CAD build for the part. Positions are in the model's coordinates, mm. Round coordinates to 2 decimals unless told otherwise and drop trailing zeros. Write each loop counter-clockwise with the first axis right and the second up, starting at its lowest first coordinate (ties: lowest second). Pieces come first, ordered by that corner, then holes. Notation, with made-up numbers: (5.25, -3.5) - (31.25, -3.5) arc R31 cw to (31.25, 34.5) - close; hole circle Ø4 at (-8.75, 86.25). An arc over 180 degrees is marked (long way). Use one line per item in the form item = value. Start each with the question number.
Item 1: Pin check, flat tip, straight feed: pin 1 (6 mm diameter, centred on x = 8, y = -19, fed in from +Z). Stop position of the tip, or through.
Item 2: Band-saw the part on C-C, the plane x = -34. List the corners of the cut face in (y, z), and give its area (3 significant figures).
Item 3: Drill centre lines: L1, parallel to X at y = -3.5, z = 9; L2, parallel to Y at x = 0.5, z = 6; L3, parallel to Z at x = -29.5, y = 23.5. Where is each one in solid material? Low to high.
Item 4: Band-saw the part on A-A, the plane z = 7.25. List the corners of the cut face in (x, y), and give its area (3 significant figures).
Item 5: Band-saw the part on B-B, the plane y = 60. List the corners of the cut face in (x, z).
from build123d import *

# Parameters (mm, degrees)
F1_W     = 83
F1_H     = 137
F2_DEPTH = 5
F0_W     = 15
F0_H     = 127
F3_DEPTH = 25
F4_R     = 2
F5_DEPTH = 5
F6_R     = 1


with BuildPart() as f2:
    # F1 (on Top) → F2 (new body, symmetric)
    with BuildSketch(Plane.XY):
        Rectangle(F1_W, F1_H)
    extrude(amount=F2_DEPTH, both=True)

    # F0 (on Top) → F3 (cut)
    with BuildSketch(Plane.XY):
        with Locations((-29, 0)):
            Rectangle(F0_W, F0_H)
        with Locations((29, 0)):
            Rectangle(F0_W, F0_H)
        with Locations((7, 0)):
            Rectangle(F0_W, F0_H)
    extrude(amount=F3_DEPTH, mode=Mode.SUBTRACT)

    # F4
    f4_edges = [f2.edges().sort_by_distance(p)[0] for p in [
        (-41.5, -68.5, 0),
        (41.5, -68.5, 0),
        (41.5, 68.5, 0),
        (-41.5, 68.5, 0),
    ]]
    fillet(f4_edges, radius=F4_R)

    # F5 (add): a face of the model
    f5_faces = [f2.faces().sort_by_distance(p)[0] for p in [
        (-2.3591054268, 0, 5),
    ]]
    extrude(f5_faces, amount=F5_DEPTH)

    # F6
    f6_edges = [f2.edges().sort_by_distance(p)[0] for p in [
        (-21.5, 0, 10),
        (-29, 63.5, 10),
        (-36.5, 0, 10),
        (-29, -63.5, 10),
        (-0.5, 0, 10),
        (14.5, 0, 10),
        (7, 63.5, 10),
        (7, -63.5, 10),
        (29, 63.5, 10),
        (21.5, 0, 10),
        (36.5, 0, 10),
        (29, -63.5, 10),
    ]]
    fillet(f6_edges, radius=F6_R)


solid = f2.part
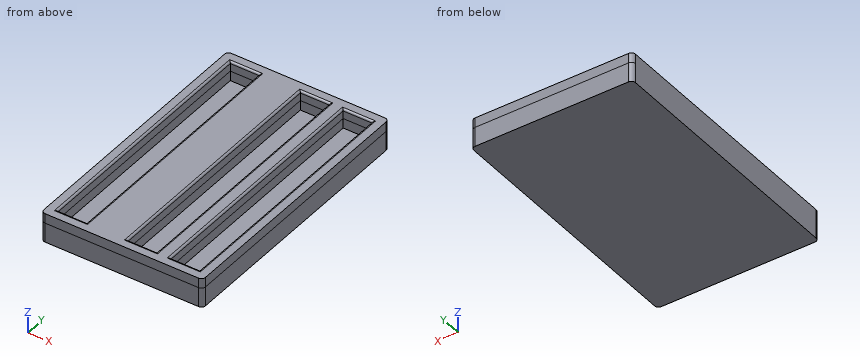
Determined:
q1.pin_1 = 0
q2.outline = (-68.5, -5) - (68.5, -5) - (68.5, 10) - (64.5, 10) arc R1 ccw to (63.5, 9) - (63.5, 0) - (-63.5, 0) - (-63.5, 9) arc R1 ccw to (-64.5, 10) - (-68.5, 10) - close
q2.area = 785 mm²
q3.L1 = -41.5 to -36.5, -21.5 to -0.5, 14.5 to 21.5, 36.5 to 41.5
q3.L2 = -68.5 to -63.5, 63.5 to 68.5
q3.L3 = -5 to 0
q4.outline = (-41.5, -66.5) arc R2 ccw to (-39.5, -68.5) - (39.5, -68.5) arc R2 ccw to (41.5, -66.5) - (41.5, 66.5) arc R2 ccw to (39.5, 68.5) - (-39.5, 68.5) arc R2 ccw to (-41.5, 66.5) - close; hole (-36.5, -63.5) - (-21.5, -63.5) - (-21.5, 63.5) - (-36.5, 63.5) - close; hole (-0.5, -63.5) - (14.5, -63.5) - (14.5, 63.5) - (-0.5, 63.5) - close; hole (21.5, -63.5) - (36.5, -63.5) - (36.5, 63.5) - (21.5, 63.5) - close
q4.area = 5,650 mm²
q5.outline = (-41.5, -5) - (41.5, -5) - (41.5, 10) - (37.5, 10) arc R1 ccw to (36.5, 9) - (36.5, 0) - (21.5, 0) - (21.5, 9) arc R1 ccw to (20.5, 10) - (15.5, 10) arc R1 ccw to (14.5, 9) - (14.5, 0) - (-0.5, 0) - (-0.5, 9) arc R1 ccw to (-1.5, 10) - (-20.5, 10) arc R1 ccw to (-21.5, 9) - (-21.5, 0) - (-36.5, 0) - (-36.5, 9) arc R1 ccw to (-37.5, 10) - (-41.5, 10) - close
